The figure shows three views and two pictorial views of one solid part (mm, origin at its lowest corner). Answer the questions. Give positions to 0.01 mm unless a question says otherwise; leave off trailing zeros. Loops run counter-clockwise (first coordinate to the right, second up) from the corner with the lowest first, then second, coordinate; pieces in that order, holes last.
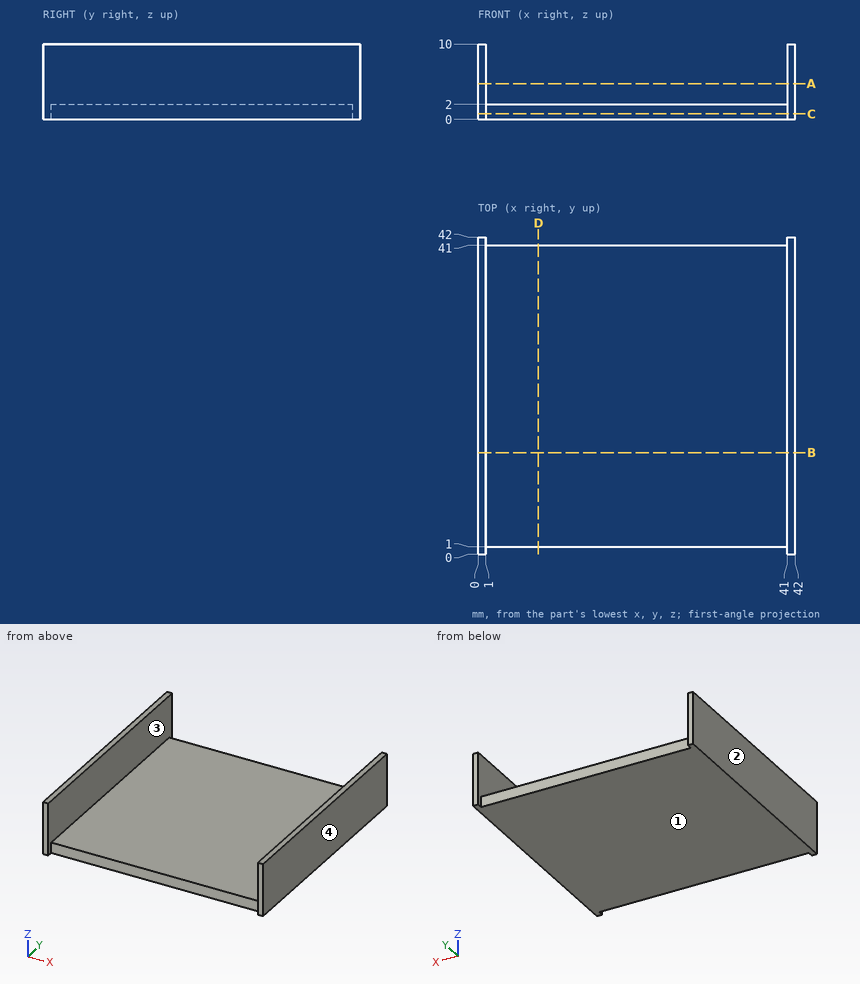
Q1. Section A-A on z = 4.75 is taken. Give the vertices of the cut face in (x, y).
Q2. Determine the mould class of the marked faces 1, 2, 3 and 4 for opening direction X: +X half, -X half, draft (parallel to the pull), parting line (faces both ways), or undercut.
Q3. Section B-B on y = 13.5 is taken. Give the vertices of the cut face in (x, z), plus the area to 3 significant figures.
Q4. Consider line 1 along X through (y, z) = (13, 3); line 2 along Z through (x, y) = (14, 22); line 3 along Y through (x, z) = (33, 1.5). Determine where each line is inside the solid, lowest interval first.
Q5. Section D-D on x = 8 is taken. Give the vertices of the cut face in (y, z), plus the area to 3 significant figures.
Q6. Given pin 1 (5 mm diameter, centred on x = 28, y = 12.5, fed in from +Z); pin 2 (2 mm diameter, centred on x = 21.5, z = 1.5, fed in from +Y); pin 3 (0.6 mm diameter, centred on x = 11.5, z = 1.5, fed in from -Y), each flat-ended and moving along its own axis, determine where each tip first touches the part or whether it passes through.
Q7. Section C-C on z = 0.75 is taken. Give the vertices of the cut face in (x, y), plus the area to 3 significant figures.
Check result:
1. outline: (0, 0) - (1, 0) - (1, 42) - (0, 42) - close; (41, 0) - (42, 0) - (42, 42) - (41, 42) - close
2. face 1: draft
2. face 2: -X half
2. face 3: undercut
2. face 4: +X half
3. outline: (0, 0) - (42, 0) - (42, 10) - (41, 10) - (41, 2) - (1, 2) - (1, 10) - (0, 10) - close
3. area: 100 mm2
4. line 1: x = 0 to 1, 41 to 42
4. line 2: z = 0 to 2
4. line 3: y = 1 to 41
5. outline: (1, 0) - (41, 0) - (41, 2) - (1, 2) - close
5. area: 80.0 mm2
6. pin 1: stops at z = 2
6. pin 2: stops at y = 41
6. pin 3: stops at y = 1
7. outline: (0, 0) - (1, 0) - (1, 1) - (41, 1) - (41, 0) - (42, 0) - (42, 42) - (41, 42) - (41, 41) - (1, 41) - (1, 42) - (0, 42) - close
7. area: 1,680 mm2
